Autodesk Inventor part; units mm, degrees
ref_plane "YZ Plane" through (0, 0, 0) normal (1, 0, 0) x (0, 1, 0)
ref_plane "XZ Plane" through (0, 0, 0) normal (0, 1, 0) x (-1, 0, 0)
ref_plane "XY Plane" through (0, 0, 0) normal (0, 0, 1) x (1, 0, 0)
sketch "Sketch1" plane through (0, 0, 0) normal (0, 1, 0) x (-1, 0, 0)
  line L0 (0, 0) -> (-60, 0)
  line L1 (-60, 0) -> (-60, -10)
  line L2 (-60, -10) -> (0, -10)
  line L3 (0, -10) -> (0, 0)
  circle A0 centre (-5, -5) radius 1.5
  circle A1 centre (-55, -5) radius 1.5
  line L4 (-30, -10) -> (-30, 0) construction
  line L5 (0, -5) -> (-5, -5) construction
  line L6 (-5, -5) -> (-30, -5) construction
  line L7 (-55, -5) -> (-60, -5) construction
  circle A2 centre (-14, -5) radius 1.5
  line L8 (-30, -5) -> (-55, -5) construction
  circle A3 centre (-46, -5) radius 1.5
  dimension "d0" = 60
  dimension "d1" = 10
  dimension "d2" = 3
  dimension "d3" = 3
  dimension "d4" = 5
  dimension "d5" = 5
  dimension "d6" = 5
  dimension "d7" = 5
  dimension "d9" = 3
  dimension "d10" = 16
extrude "Extrusion1" add sketch "Sketch1" along normal blind 5
chamfer "Chamfer1" distance 2.5 angle 45 2 edges at (0, 2.5, 0) (60, 2.5, 0)
fillet "Fillet1" radius 1 12 edges at (30, 5, 0) (1.25, 5, -1.25) (0, 5, -6.25) (0, 2.5, -2.5) (2.5, 2.5, 0) (57.5, 2.5, 0) (58.75, 5, -1.25) (60, 2.5, -2.5) (60, 5, -6.25) (60, 2.5, -10) (0, 2.5, -10) (30, 5, -10)
equation "\"d3\" = d2"
equation "\"d5\" = d4"
equation "\"d6\" = 0.5 * d1"
equation "\"d7\" = d6"
equation "\"d9\" = d2"
properties part number "fan_duct_holder"
Check sheet for the modelled part. Datum: model origin and axes. Units: mm. Round coordinates to 2 decimals unless told otherwise and drop trailing zeros. Order: outer loops, then holes, each group sorted by start corner. A loop starts at its lowest first (then second) coordinate and runs counter-clockwise, first axis right, second up.
Q1. Scan lines: L1, parallel to Z at x = 5, y = 3.9; L2, parallel to X at y = 3.2, z = -4.75; L3, parallel to Z at x = 14.5, y = 3.3. Record each from-to range of solid material in increasing order.
Filled sheet:
L1: z = -10 to -6.5, -3.5 to 0
L2: x = 0 to 3.52, 6.48 to 12.52, 15.48 to 44.52, 47.48 to 53.52, 56.48 to 60
L3: z = -10 to -6.41, -3.59 to 0
Q2. Cross-section at B-B, the plane z = -5. Enter the section's corners in (x, y).
Filled sheet:
outline: (0, 0) - (3.5, 0) - (3.5, 5) - (1, 5) arc R1 ccw to (0, 4) - close; (6.5, 0) - (12.5, 0) - (12.5, 5) - (6.5, 5) - close; (15.5, 0) - (44.5, 0) - (44.5, 5) - (15.5, 5) - close; (47.5, 0) - (53.5, 0) - (53.5, 5) - (47.5, 5) - close; (56.5, 0) - (60, 0) - (60, 4) arc R1 ccw to (59, 5) - (56.5, 5) - close
Q3. Cross-section at D-D, the plane x = 55.5. Enter the section's corners in (y, z).
Filled sheet:
outline: (0, -10) - (4, -10) arc R1 ccw to (5, -9) - (5, -6.41) - (0, -6.41) - close; (0, -3.59) - (5, -3.59) - (5, -1) arc R1 ccw to (4, 0) - (0, 0) - close
Q4. Cross-section at A-A, the plane x = 5. Enter the section's corners in (y, z), plus the area to 3 significant figures.
Filled sheet:
outline: (0, -10) - (4, -10) arc R1 ccw to (5, -9) - (5, -6.5) - (0, -6.5) - close; (0, -3.5) - (5, -3.5) - (5, -1) arc R1 ccw to (4, 0) - (0, 0) - close
area: 34.6 mm2
Q5. Cross-section at C-C, the plane y = 1. Enter the section's corners in (x, z).
Filled sheet:
outline: (0, -9) arc R1 ccw to (1, -10) - (59, -10) arc R1 ccw to (60, -9) - (60, -2.91) arc R1 ccw to (59.71, -2.21) - (57.79, -0.29) arc R1 ccw to (57.09, 0) - (2.91, 0) arc R1 ccw to (2.21, -0.29) - (0.29, -2.21) arc R1 ccw to (0, -2.91) - close; hole circle Ø3 at (5, -5); hole circle Ø3 at (14, -5); hole circle Ø3 at (46, -5); hole circle Ø3 at (55, -5)
Q6. Depth check by flat-ended pin: P1, Ø5, axis at x = 5, z = -5, coming from the +Y side. Enter the tip coordinate at first touch or a pass-through.
Filled sheet:
P1: stops at y = 5
Q7. Draft check along X on faces 1 (the face through (53.57, 2.46, -5.45)), 2 (the face through (30, 2, 0)), 3 (the face through (6.2, 2.5, -4.1)), 4 (the face through (59.715, 2.028, -9.699)). Enter one of: pulls with the +X half, pulls with the -X half, needs draft (parallel to the pull), parting line crosses it, or undercut.
Filled sheet:
face 1: undercut
face 2: needs draft
face 3: undercut
face 4: pulls with the +X half
